Source: three-view drawing plus pictorial views. Frame: mm from the lowest corner of the part. A direction names the side the tool comes from. Give positions to 0.01 mm unless a question says otherwise; leave off trailing zeros. Loops run counter-clockwise (first coordinate to the right, second up) from the corner with the lowest first, then second, coordinate; pieces in that order, holes last.
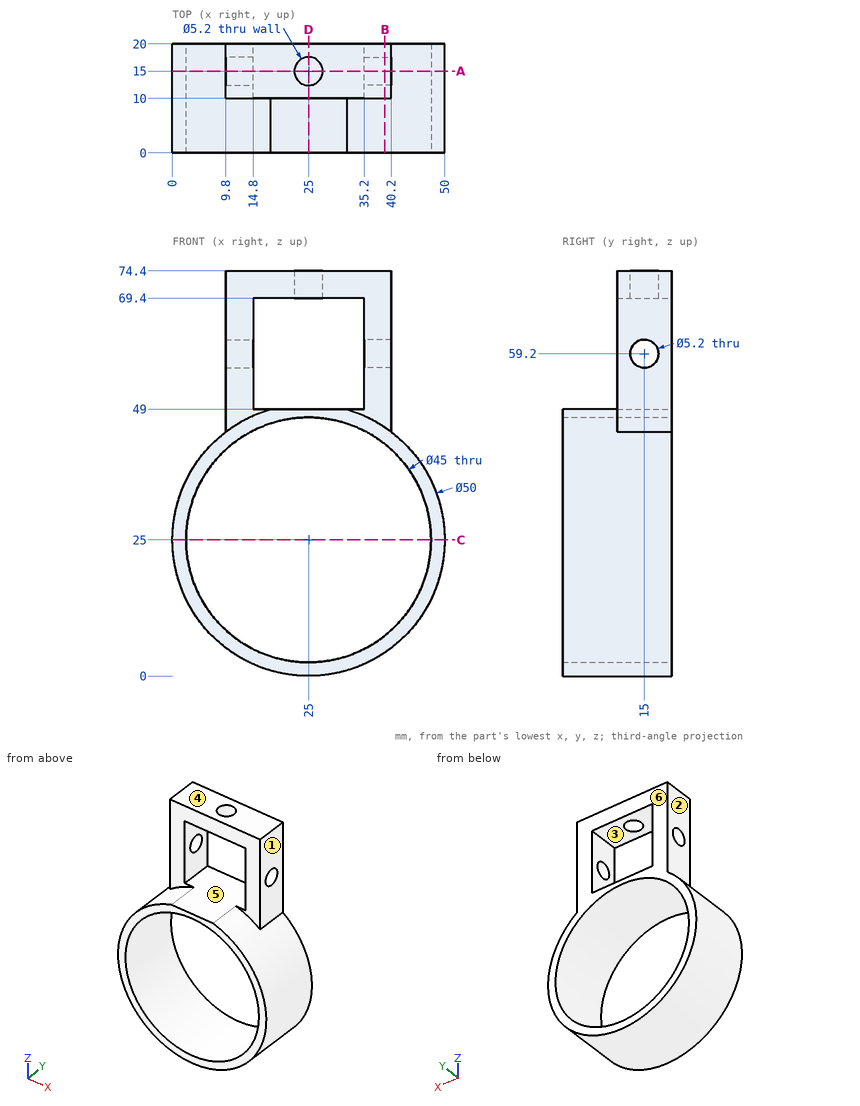
Q1. Mould query, pull axis Z, two halves, no side actions, for the marked faces 4, 5 and 6. Classes: +Z half, -Z half, draft (parallel to the pull), parting line (faces both ways), or undercut.
Q2. Section query C-C, the plane z = 25. Return loops of the section in (x, y), and give its area (3 significant figures).
Q3. Section query D-D, the plane x = 25. Return loops of the section in (y, z).
Q4. Section query A-A, the plane y = 15. Return loops of the section in (x, z), and give its area (3 significant figures).
Q5. Material intervals for probe 1 along Z at (x, y) = (16, 11); probe 2 along X at (y, z) = (16, 25); probe 3 along Y at (x, z) = (39, 59), sorted ascending.
Q6. Pin query (flat end, axial travel): pin 1 Ø1.5 at (x, y) = (34.5, 17) entering from -Z; pin 2 Ø2 at (y, z) = (16, 39) entering from -X; pin 3 Ø5 at (x, y) = (41, 9) entering from -Z. Return the tip coordinate at first contact, or that it passes through.
Q7. Reachability of the marked faces 1, 2 and 3 from +Z, -Z, +X, -X, +Y, -Y: full face, straight path, thin tool, end or side. Return the list, or none.
Q8. Section query B-B, the plane x = 39. Return loops of the section in (y, z), and give its area (3 significant figures).
Resolved:
1. face 4: +Z half
1. face 5: undercut
1. face 6: draft
2. outline: (0, 0) - (2.5, 0) - (2.5, 20) - (0, 20) - close; (47.5, 0) - (50, 0) - (50, 20) - (47.5, 20) - close
2. area: 100 mm2
3. outline: (0, 0) - (20, 0) - (20, 2.5) - (0, 2.5) - close; (0, 47.5) - (20, 47.5) - (20, 49) - (0, 49) - close; (10, 69.4) - (12.4, 69.4) - (12.4, 74.4) - (10, 74.4) - close; (17.6, 69.4) - (20, 69.4) - (20, 74.4) - (17.6, 74.4) - close
4. outline: (9.8, 44.85) arc R25 ccw (long way) to (40.2, 44.85) - (40.2, 56.6) - (35.2, 56.6) - (35.2, 49) - (14.8, 49) - (14.8, 56.6) - (9.8, 56.6) - close; (9.8, 61.8) - (14.8, 61.8) - (14.8, 69.4) - (22.4, 69.4) - (22.4, 74.4) - (9.8, 74.4) - close; (27.6, 69.4) - (35.2, 69.4) - (35.2, 61.8) - (40.2, 61.8) - (40.2, 74.4) - (27.6, 74.4) - close; hole circle Ø45 at (25, 25)
4. area: 671 mm2
5. probe 1: z = 1.68 to 4.38, 45.62 to 49, 69.4 to 74.4
5. probe 2: x = 0 to 2.5, 47.5 to 50
5. probe 3: y = 10 to 12.41, 17.59 to 20
6. pin 1: stops at z = 1.58
6. pin 2: stops at x = 3.65
6. pin 3: stops at z = 3.96
7. face 1: +Z, +X, +Y, -Y
7. face 2: +Z, -X, +Y, -Y
7. face 3: +Y, -Y
8. outline: (0, 4.29) - (20, 4.29) - (20, 7.39) - (0, 7.39) - close; (0, 42.61) - (20, 42.61) - (20, 74.4) - (10, 74.4) - (10, 45.71) - (0, 45.71) - close; hole circle Ø5.2 at (15, 59.2)
8. area: 390 mm2
